The listing builds one solid part. Answer for the finished solid, in the listing's coordinates (mm). Coordinates: 2 decimals unless noted, no trailing zeros. Order: outer loops, then holes, each group sorted by start corner. A loop starts at its lowest first (then second) coordinate and runs counter-clockwise, first axis right, second up. Notation, with made-up numbers: (30.5, -3.75) -> (38.5, -3.75) arc R22 cw to (38.5, 31.25) -> close; hole circle Ø9 at (67.5, 58). An arc over 180 degrees is marked (long way). One line per question, with ' | ' between items.
Autodesk Inventor part; units mm, degrees
ref_plane "1_XY" through (0, 0, 0) normal (1, 0, 0) x (0, 0, -1)
ref_plane "1_YZ" through (0, 0, 0) normal (0, 0, -1) x (0, 1, 0)
ref_plane "1_ZX" through (0, 0, 0) normal (0, 1, 0) x (1, 0, 0)
sketch "Sketch_5" plane through (0, 0, 0) normal (1, 0, 0) x (0, 1, 0)
  arc A0 (-2.3939, -2.2747) -> (-2.3939, 2.2747) centre (0.2, 0) ccw
  arc A1 (-3.2209, 1.9) -> (-2.3939, 2.2747) centre (-3.2209, 3) ccw
  line L0 (-3.2209, 1.9) -> (-3.75, 1.9)
  arc A2 (-3.75, 1.9) -> (-4.85, 0.8) centre (-3.75, 0.8) ccw
  line L1 (-4.85, 0.8) -> (-4.85, 0.025)
  line L2 (-4.85, 0.025) -> (-4.1, 0.025)
  line L3 (-4.1, 0.025) -> (-4.1, 0.7)
  arc A3 (-3.4, 0.7) -> (-4.1, 0.7) centre (-3.75, 0.7) ccw
  line L4 (-3.4, 0.7) -> (-3.4, 0.025)
  line L5 (-3.4, 0.025) -> (-2.8499, 0.025)
  arc A4 (-2.8499, -0.025) -> (-2.8499, 0.025) centre (0, 0) ccw
  line L6 (-2.8499, -0.025) -> (-3.4, -0.025)
  line L7 (-3.4, -0.025) -> (-3.4, -0.7)
  arc A5 (-4.1, -0.7) -> (-3.4, -0.7) centre (-3.75, -0.7) ccw
  line L8 (-4.1, -0.7) -> (-4.1, -0.025)
  line L9 (-4.1, -0.025) -> (-4.85, -0.025)
  line L10 (-4.85, -0.025) -> (-4.85, -0.8)
  arc A6 (-4.85, -0.8) -> (-3.75, -1.9) centre (-3.75, -0.8) ccw
  line L11 (-3.75, -1.9) -> (-3.2209, -1.9)
  arc A7 (-2.3939, -2.2747) -> (-3.2209, -1.9) centre (-3.2209, -3) ccw
extrude "Extrusion1" add sketch "Sketch_5" along normal mid plane 0.4
ref_plane "1_XY" through (0, 0, 0) normal (1, 0, 0) x (0, 0, -1)
ref_plane "1_YZ" through (0, 0, 0) normal (0, 0, -1) x (0, 1, 0)
ref_plane "1_ZX" through (0, 0, 0) normal (0, 1, 0) x (1, 0, 0)
ref_plane "combination_module_XY" through (0.2, 0, 0) normal (1, 0, 0) x (0, 0, -1)
ref_plane "combination_module_YZ" through (0.2, 0, 0) normal (0, 0, -1) x (0, 1, 0)
ref_plane "combination_module_ZX" through (0.2, 0, 0) normal (0, 1, 0) x (1, 0, 0)
properties part number "SL-STWS6"
Item 1: Section A-A, the plane z = 0.5 is taken. Give the vertices of the cut face in (x, y), plus the area to 3 significant figures.
Computed values:
outline: (-0.2, -4.85) -> (0.2, -4.85) -> (0.2, -4.1) -> (-0.2, -4.1) -> close; (-0.2, -3.4) -> (0.2, -3.4) -> (0.2, -2.81) -> (-0.2, -2.81) -> close; (-0.2, 2.81) -> (0.2, 2.81) -> (0.2, 3.61) -> (-0.2, 3.61) -> close | area: 0.861 mm^2
Item 2: Section B-B, the plane y = -1.25 is taken. Give the vertices of the cut face in (x, z), plus the area to 3 significant figures.
Computed values:
outline: (-0.2, -3.13) -> (0.2, -3.13) -> (0.2, -2.56) -> (-0.2, -2.56) -> close; (-0.2, 2.56) -> (0.2, 2.56) -> (0.2, 3.13) -> (-0.2, 3.13) -> close | area: 0.455 mm^2
Item 3: Section D-D, the plane z = -0.25 is taken. Give the vertices of the cut face in (x, y), plus the area to 3 significant figures.
Computed values:
outline: (-0.2, -4.85) -> (0.2, -4.85) -> (0.2, -4.1) -> (-0.2, -4.1) -> close; (-0.2, -3.4) -> (0.2, -3.4) -> (0.2, -2.84) -> (-0.2, -2.84) -> close; (-0.2, 2.84) -> (0.2, 2.84) -> (0.2, 3.64) -> (-0.2, 3.64) -> close | area: 0.845 mm^2
Item 4: Find the intervals of material crossed by L1, parallel to Y at x = -0.05, z = -0.75; L2, parallel to Y at x = -0.05, z = 0.5; L3, parallel to Z at x = 0.1, y = -1, in increasing order.
Computed values:
L1: y = -4.85 to -4.1, -3.4 to -2.75, 2.75 to 3.57 | L2: y = -4.85 to -4.1, -3.4 to -2.81, 2.81 to 3.61 | L3: z = -3.23 to -2.67, 2.67 to 3.23
Item 5: Determine the mould class of faces 1 (the face through (-0.003, -4.536, 1.569)), 2 (the face through (-0.003, 2.847, 0.125)), 3 (the face through (-0.2, -3, 1)) for opening direction Z: pulls with the +Z half, pulls with the -Z half, needs draft (parallel to the pull), parting line crosses it, or undercut.
Computed values:
face 1: pulls with the +Z half | face 2: undercut | face 3: needs draft
Item 6: Section C-C, the plane x = -0.1 is taken. Give the vertices of the cut face in (y, z) (3 decimals), plus the area to 3 significant figures.
Computed values:
outline: (-4.85, -0.8) arc R1.1 ccw to (-3.75, -1.9) -> (-3.221, -1.9) arc R1.1 cw to (-2.394, -2.275) arc R3.45 ccw (long way) to (-2.394, 2.275) arc R1.1 cw to (-3.221, 1.9) -> (-3.75, 1.9) arc R1.1 ccw to (-4.85, 0.8) -> (-4.85, 0.025) -> (-4.1, 0.025) -> (-4.1, 0.7) arc R0.35 cw to (-3.4, 0.7) -> (-3.4, 0.025) -> (-2.85, 0.025) arc R2.85 cw (long way) to (-2.85, -0.025) -> (-3.4, -0.025) -> (-3.4, -0.7) arc R0.35 cw to (-4.1, -0.7) -> (-4.1, -0.025) -> (-4.85, -0.025) -> close | area: 16.8 mm^2
